CAD build for the part. Positions are in the model's coordinates, mm. Give positions to 0.01 mm unless a question says otherwise; leave off trailing zeros. Order: outer loops, then holes, each group sorted by start corner. A loop starts at its lowest first (then second) coordinate and runs counter-clockwise, first axis right, second up. Notation, with made-up numbers: M 50,68 L 94,68 A6 cw 94,72 Z; hole C -11,-7 d2. An arc over 180 degrees is marked long. Put each result on its own line as item: value. Start each with the question number.
1) Drill centre lines: line 1 (X direction, y = 1.55, z = 4); line 2 (Z direction, x = -52.5, y = 1.2); line 3 (X direction, y = 1.05, z = -3.25). Where is each one in solid material? Low to high. Write a range as [from, to].
2) Cut at A-A (x = 24.75). Write the cut outline in (y, z) (3 decimals), and give its area (3 significant figures).
3) Two-plate mould, pull along X, no slides. Class faces 1 (the face through (-57.5, 1, 0)), 2 (the face through (-1, 1, -7.5)), 3 (the face through (-38.253, 0.974, -0.132)), 4 (the face through (-11.02, 0.97, 1.15)): released by +X, released by -X, zero draft, split by the parting line, or undercut.
4) Cut at B-B (y = 0.9). Give the number of separate pieces and of enclosed holes in the cut face, and give its area (3 significant figures).
5) Cut at C-C (x = 52.5). Write the cut outline in (y, z) (3 decimals), and give its area (3 significant figures).
```python
from build123d import *

# Parameters (mm, degrees)
SKETCH1_W                            = 115
SKETCH1_H                            = 15
BOSS_EXTRUDE1_DEPTH                  = 2
F_3_3_3_3_DIAMETER_HOLE1_D           = 3.3
F_3_3_3_3_DIAMETER_HOLE1_DEPTH       = 15
F_3_3_3_3_DIAMETER_HOLE1_CSINK_D     = 3.35
F_3_3_3_3_DIAMETER_HOLE1_CSINK_ANGLE = 90
F_3_3_3_3_DIAMETER_HOLE1_TIP         = 0.991420021
F_6_0_6_DIAMETER_HOLE1_D             = 6
F_6_0_6_DIAMETER_HOLE1_DEPTH         = 15
F_6_0_6_DIAMETER_HOLE1_CSINK_D       = 6.05
F_6_0_6_DIAMETER_HOLE1_CSINK_ANGLE   = 90
F_6_0_6_DIAMETER_HOLE1_TIP           = 1.802581857


with BuildPart() as part:
    # Sketch1 → Boss-Extrude1 (new body)
    with BuildSketch(Plane(origin=(0, 0, 0), x_dir=(1, 0, 0), z_dir=(0, 1, 0))):
        Rectangle(SKETCH1_W, SKETCH1_H)
    extrude(amount=BOSS_EXTRUDE1_DEPTH)

    # Ø3.3 (3.3) Diameter Hole1
    with Locations(Plane(origin=(0, 2, 0), x_dir=(1, 0, 0), z_dir=(0, 1, 0))):
        with Locations((52.5, -4), (-52.5, 4), (-52.5, -4), (52.5, 4)):
            CounterSinkHole(F_3_3_3_3_DIAMETER_HOLE1_D / 2, F_3_3_3_3_DIAMETER_HOLE1_CSINK_D / 2, depth=F_3_3_3_3_DIAMETER_HOLE1_DEPTH, counter_sink_angle=F_3_3_3_3_DIAMETER_HOLE1_CSINK_ANGLE)
            with Locations((0, 0, -(F_3_3_3_3_DIAMETER_HOLE1_DEPTH + F_3_3_3_3_DIAMETER_HOLE1_TIP / 2))):  # 118° drill point
                Cone(0, F_3_3_3_3_DIAMETER_HOLE1_D / 2, F_3_3_3_3_DIAMETER_HOLE1_TIP, mode=Mode.SUBTRACT)

    # Ø6.0 (6) Diameter Hole1
    with Locations(Plane(origin=(0, 2, 0), x_dir=(1, 0, 0), z_dir=(0, 1, 0))):
        with Locations((-8.25, 0), (8.25, 0), (24.75, 0), (41.25, 0), (-24.75, 0), (-41.25, 0)):
            CounterSinkHole(F_6_0_6_DIAMETER_HOLE1_D / 2, F_6_0_6_DIAMETER_HOLE1_CSINK_D / 2, depth=F_6_0_6_DIAMETER_HOLE1_DEPTH, counter_sink_angle=F_6_0_6_DIAMETER_HOLE1_CSINK_ANGLE)
            with Locations((0, 0, -(F_6_0_6_DIAMETER_HOLE1_DEPTH + F_6_0_6_DIAMETER_HOLE1_TIP / 2))):  # 118° drill point
                Cone(0, F_6_0_6_DIAMETER_HOLE1_D / 2, F_6_0_6_DIAMETER_HOLE1_TIP, mode=Mode.SUBTRACT)


solid = part.part
```
Solution:
1. line 1: [-57.5, -54.15], [-50.85, 50.85], [54.15, 57.5]
1. line 2: [-7.5, -5.65], [-2.35, 2.35], [5.65, 7.5]
1. line 3: [-57.5, -53.97], [-51.03, 51.03], [53.97, 57.5]
2. outline: M 0,-7.5 L 2,-7.5 L 2,-3.025 L 1.975,-3 L 0,-3 Z; M 0,3 L 1.975,3 L 2,3.025 L 2,7.5 L 0,7.5 Z
2. area: 18.0 mm²
3. face 1: released by -X
3. face 2: zero draft
3. face 3: undercut
3. face 4: undercut
4. separate pieces: 1
4. enclosed holes: 10
4. area: 1,520 mm²
5. outline: M 0,-7.5 L 2,-7.5 L 2,-5.675 L 1.975,-5.65 L 0,-5.65 Z; M 0,-2.35 L 1.975,-2.35 L 2,-2.325 L 2,2.325 L 1.975,2.35 L 0,2.35 Z; M 0,5.65 L 1.975,5.65 L 2,5.675 L 2,7.5 L 0,7.5 Z
5. area: 16.8 mm²
